Part model, mm, in its own coordinate system. Face numbers are marked on the shaded views. Coordinates: 2 decimals unless noted, no trailing zeros. Write each loop counter-clockwise with the first axis right and the second up, starting at its lowest first coordinate (ties: lowest second). Pieces come first, ordered by that corner, then holes. Notation, with made-up numbers: (66, 50) -> (108, 50) arc R28 cw to (108, 76) -> close; hole circle Ø9 at (-1.5, 50). An arc over 180 degrees is marked (long way). Write item = value, one per line. Start each with the question number.
Q1. Band-saw the part on C-C, the plane z = 13. List the corners of the cut face in (x, y) (3 decimals).
Q2. Band-saw the part on B-B, the plane x = 0. List the corners of the cut face in (y, z), plus the area to 3 significant figures.
Q3. Probe line 1 (Y direction, x = 0, z = 4.25); line 2 (X direction, y = -40, z = 17.5); line 3 (X direction, y = 12.5, z = 5.75). List the from-to ranges inside material, lowest first.
Q4. Band-saw the part on D-D, the plane y = -107.95. List the corners of the cut face in (x, z).
Q5. Band-saw the part on A-A, the plane y = 0. List the corners of the cut face in (x, z).
Q6. Pin check, flat tips, straight feed: P1, Ø5.5, axis at x = 93.49, y = -53.98, coming from the +Z side; P2, Ø4, axis at y = -75, z = 11, coming from the -X side; P3, Ø10, axis at y = 8.5, z = 5.5, coming from the +X side; P4, Ø1, axis at x = 76.5, z = 6, coming from the +Y side. Stop position of each tip, or through.
Q7. Pull direction X, two halves, no side cores. Call the marked faces 1, 2 and 3: released by +X, released by -X, zero draft, split by the parting line, or undercut.
from build123d import *

# Parameters (mm, degrees)
SKETCH1_R               = 127
BOSS_EXTRUDE1_DEPTH     = 19.05
F_1_4_CLEARANCE_HOLE1_D = 7.14248
CUT_EXTRUDE1_REACH      = 182.613
SKETCH4_R               = 63.5


with BuildPart() as part:
    # Sketch1 → Boss-Extrude1 (new body)
    with BuildSketch(Plane.XY):
        with Locations(Location((0, 0, 0), (0, 0, 180))):
            Circle(SKETCH1_R)
    extrude(amount=BOSS_EXTRUDE1_DEPTH)

    # 1/4 Clearance Hole1 (through all)
    with Locations(Plane.XY.offset(19.05)):
        with Locations((-93.487442339, 53.975), (0, 107.95), (93.487442339, 53.975), (93.487442339, -53.975), (0, -107.95), (-93.487442339, -53.975)):
            Hole(F_1_4_CLEARANCE_HOLE1_D / 2)

    # Sketch4 → Cut-Extrude1 (cut, up to next)
    with BuildSketch(Plane.XY.offset(19.05), mode=Mode.PRIVATE) as cut_extrude1_sk1:
        Circle(SKETCH4_R)
    cut_extrude1_tool1 = extrude(cut_extrude1_sk1.sketch, amount=-CUT_EXTRUDE1_REACH, mode=Mode.PRIVATE) & part.part
    add(cut_extrude1_tool1.solids().sort_by_distance((0, 0, 19.05))[0], mode=Mode.SUBTRACT)


solid = part.part
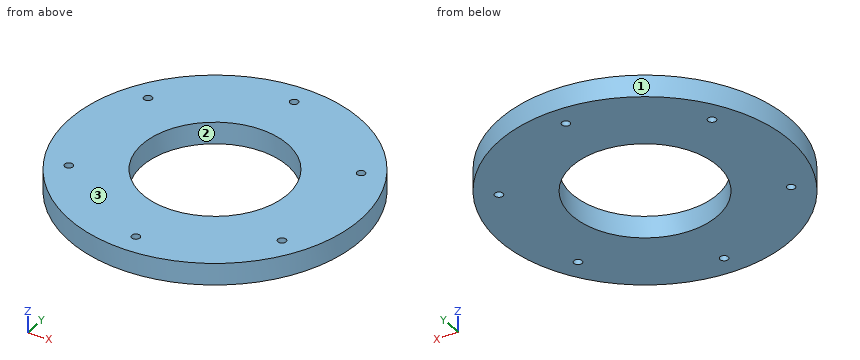
Ans:
q1.outline = circle Ø254 at (0, 0); hole circle Ø7.142 at (-93.487, -53.975); hole circle Ø7.142 at (-93.487, 53.975); hole circle Ø127 at (0, 0); hole circle Ø7.142 at (0, -107.95); hole circle Ø7.142 at (0, 107.95); hole circle Ø7.142 at (93.487, -53.975); hole circle Ø7.142 at (93.487, 53.975)
q2.outline = (-127, 0) -> (-111.52, 0) -> (-111.52, 19.05) -> (-127, 19.05) -> close; (-104.38, 0) -> (-63.5, 0) -> (-63.5, 19.05) -> (-104.38, 19.05) -> close; (63.5, 0) -> (104.38, 0) -> (104.38, 19.05) -> (63.5, 19.05) -> close; (111.52, 0) -> (127, 0) -> (127, 19.05) -> (111.52, 19.05) -> close
q2.area = 2,150 mm2
q3.line_1 = -127 to -111.52, -104.38 to -63.5, 63.5 to 104.38, 111.52 to 127
q3.line_2 = -120.54 to -49.32, 49.32 to 120.54
q3.line_3 = -126.38 to -62.26, 62.26 to 126.38
q4.outline = (-66.9, 0) -> (-3.57, 0) -> (-3.57, 19.05) -> (-66.9, 19.05) -> close; (3.57, 0) -> (66.9, 0) -> (66.9, 19.05) -> (3.57, 19.05) -> close
q5.outline = (-127, 0) -> (-63.5, 0) -> (-63.5, 19.05) -> (-127, 19.05) -> close; (63.5, 0) -> (127, 0) -> (127, 19.05) -> (63.5, 19.05) -> close
q6.P1 = through
q6.P2 = -103.92
q6.P3 = 126.95
q6.P4 = 101.75
q7.face_1 = split by the parting line
q7.face_2 = undercut
q7.face_3 = zero draft
